```python
from build123d import *

# Parameters (mm, degrees)
F0_R     = 2.125
F1_DEPTH = 2.5


with BuildPart() as f1:
    # F0 (on Top) → F1 (new body, symmetric)
    with BuildSketch(Plane.XY):
        with BuildLine():
            Line((-134.7, -107.95), (134.7, -107.95))
            ThreePointArc((134.7, -107.95), (138.235534, -106.485534), (139.7, -102.95))
            Line((139.7, -102.95), (139.7, 0))
            Line((139.7, 0), (139.7, 102.95))
            ThreePointArc((139.7, 102.95), (138.235534, 106.485534), (134.7, 107.95))
            Line((134.7, 107.95), (-134.7, 107.95))
            ThreePointArc((-134.7, 107.95), (-138.235534, 106.485534), (-139.7, 102.95))
            Line((-139.7, 102.95), (-139.7, 0))
            Line((-139.7, 0), (-139.7, -102.95))
            ThreePointArc((-139.7, -102.95), (-138.235534, -106.485534), (-134.7, -107.95))
        make_face()
        with Locations((-104.5, -104.5)):
            Circle(F0_R, mode=Mode.SUBTRACT)
        with Locations((-69.5, -44.5)):
            Circle(F0_R, mode=Mode.SUBTRACT)
        with Locations((-39.5, -44.5)):
            Circle(F0_R, mode=Mode.SUBTRACT)
        with Locations((104.5, -104.5)):
            Circle(F0_R, mode=Mode.SUBTRACT)
        with Locations((39.5, -44.5)):
            Circle(F0_R, mode=Mode.SUBTRACT)
        with Locations((69.5, -44.5)):
            Circle(F0_R, mode=Mode.SUBTRACT)
        with Locations((0, -24)):
            Circle(F0_R, mode=Mode.SUBTRACT)
        with Locations((0, -9)):
            Circle(F0_R, mode=Mode.SUBTRACT)
        with BuildLine():
            ThreePointArc((-119.7, 37.5), (-113.689592, 35.010408), (-111.2, 29))
            Line((-111.2, 29), (-111.2, -29))
            ThreePointArc((-111.2, -29), (-113.689592, -35.010408), (-119.7, -37.5))
            ThreePointArc((-119.7, -37.5), (-125.710408, -35.010408), (-128.2, -29))
            Line((-128.2, -29), (-128.2, 29))
            ThreePointArc((-128.2, 29), (-125.710408, 35.010408), (-119.7, 37.5))
        make_face(mode=Mode.SUBTRACT)
        with Locations((-69.5, 44.5)):
            Circle(F0_R, mode=Mode.SUBTRACT)
        with Locations((-39.5, 44.5)):
            Circle(F0_R, mode=Mode.SUBTRACT)
        with Locations((-104.5, 104.5)):
            Circle(F0_R, mode=Mode.SUBTRACT)
        with Locations((0, 9)):
            Circle(F0_R, mode=Mode.SUBTRACT)
        with Locations((0, 24)):
            Circle(F0_R, mode=Mode.SUBTRACT)
        with Locations((39.5, 44.5)):
            Circle(F0_R, mode=Mode.SUBTRACT)
        with Locations((69.5, 44.5)):
            Circle(F0_R, mode=Mode.SUBTRACT)
        with Locations((0, 104.5)):
            Circle(F0_R, mode=Mode.SUBTRACT)
        with Locations((104.5, 104.5)):
            Circle(F0_R, mode=Mode.SUBTRACT)
    extrude(amount=F1_DEPTH, both=True)


solid = f1.part
```
The model under review builds one solid part; all positions refer to its coordinate system, in mm. Give positions to 0.01 mm unless a question says otherwise; leave off trailing zeros. Answer in a Markdown table with one row per item.
Item 1: For line 1 along Y through (x, z) = (0, -1) (3 decimals); line 2 along X through (y, z) = (-9.5, 0.55); line 3 along Y through (x, z) = (-69.5, -0.2) (3 decimals), list the stretches that pass through material, from the lowest coordinate up.
Check sheet entries:
| item | result |
|---|---|
| line 1 | -107.95 to -26.125, -21.875 to -11.125, -6.875 to 6.875, 11.125 to 21.875, 26.125 to 102.375, 106.625 to 107.95 |
| line 2 | -139.7 to -128.2, -111.2 to -2.07, 2.07 to 139.7 |
| line 3 | -107.95 to -46.625, -42.375 to 42.375, 46.625 to 107.95 |
Item 2: For P1, Ø3.5, axis at x = 0, y = 104.5, coming from the -Z side, flat-tipped, find the tip position at first contact; note if it passes through.
Check sheet entries:
| item | result |
|---|---|
| P1 | through |
Item 3: Add section A-A on z = 1.6. State how many separate pieces and enclosed holes the cut face has, plus the area to 3 significant figures.
Check sheet entries:
| item | result |
|---|---|
| separate pieces | 1 |
| enclosed holes | 18 |
| area | 58,800 mm2 |
